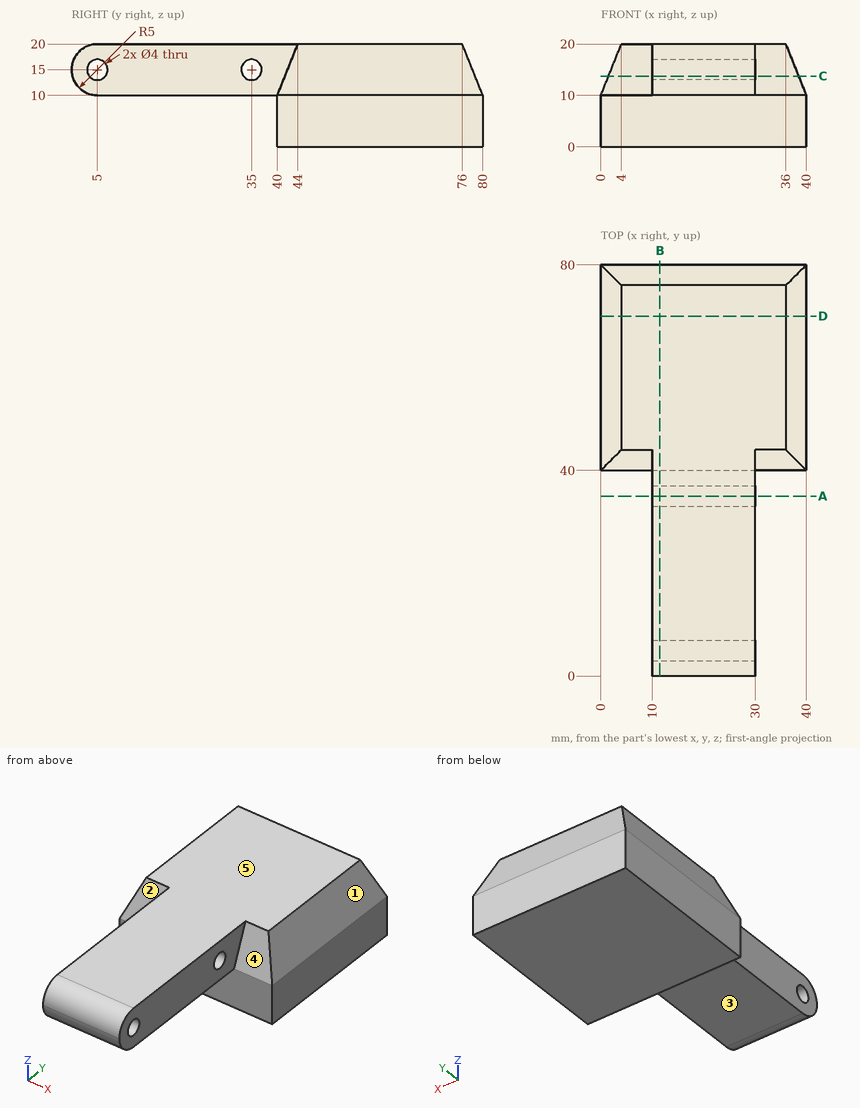
Can you work these out from the drawing? Everything is in mm from the part's minimum corner. A direction names the side the tool comes from. Give positions to 0.01 mm unless a question says otherwise; leave off trailing zeros. Order: outer loops, then holes, each group sorted by start corner. A loop starts at its lowest first (then second) coordinate and runs counter-clockwise, first axis right, second up. Notation, with made-up numbers: M -10.75,19 L 32.25,19 A20 cw 32.25,32 Z; hole C 39.25,78 d9. An arc over 180 degrees is marked long. Use a Markdown table: item, result. Add a question column.
1. For pin 1 Ø22 at (x, y) = (21, 22.5) entering from -Z; pin 2 Ø8 at (y, z) = (30, 17) entering from +X; pin 3 Ø3 at (y, z) = (27, 16) entering from -X, each with a flat end and sliding along its axis, tell me the tip position at first contact or that it passes through.
2. Suppose I cut it at C-C (z = 13.75). List the corners of the cut face in (x, y) for me, and give its area (3 significant figures).
3. I need wall thicknesses on probe 1 along Y at (x, z) = (10.5, 14.25); probe 2 along Y at (x, z) = (16.5, 15); probe 3 along Y at (x, z) = (9, 2). Which ranges of each line are inside material? Lowest first, please. Write a range as from..to.
4. On a 3-axis mill with a long thin cutter (end or side, diameter ignored), from which of +Z, -Z, +X, -X, +Y, -Y can I reach the whole of each face in a straight line? I mean the marked faces 1, 2, 3, 4 and 5. Say none if no direction works.
5. Suppose I cut it at D-D (y = 70). List the corners of the cut face in (x, z) for me.
6. Suppose I cut it at B-B (x = 11.5). List the corners of the cut face in (y, z) for me.
7. Suppose I cut it at A-A (y = 35). List the corners of the cut face in (x, z) for me.
Results list:
| question | item | result |
|---|---|---|
| 1 | pin 1 | stops at z = 10 |
| 1 | pin 2 | stops at x = 30 |
| 1 | pin 3 | stops at x = 10 |
| 2 | outline | M 1.5,41.5 L 10,41.5 L 10,36.56 L 30,36.56 L 30,41.5 L 38.5,41.5 L 38.5,78.5 L 1.5,78.5 Z; M 10,0.16 L 30,0.16 L 30,3.44 L 10,3.44 Z; M 10,6.56 L 30,6.56 L 30,33.44 L 10,33.44 Z |
| 2 | area | 2,070 mm² |
| 3 | probe 1 | y = 0.06..3.15, 6.85..33.15, 36.85..78.3 |
| 3 | probe 2 | y = 0..3, 7..33, 37..78 |
| 3 | probe 3 | y = 40..80 |
| 4 | face 1 | +Z, +X, +Y, -Y |
| 4 | face 2 | +Z, -X, -Y |
| 4 | face 3 | -Z, +X, -X, -Y |
| 4 | face 4 | +Z, +X, -Y |
| 4 | face 5 | +Z, +X, -X, +Y, -Y |
| 5 | outline | M 0,0 L 40,0 L 40,10 L 36,20 L 4,20 L 0,10 Z |
| 6 | outline | M 5,10 L 40,10 L 40,0 L 80,0 L 80,10 L 76,20 L 5,20 A5 ccw Z; hole C 5,15 d4; hole C 35,15 d4 |
| 7 | outline | M 10,10 L 30,10 L 30,13 L 10,13 Z; M 10,17 L 30,17 L 30,20 L 10,20 Z |
